Verification items for the finished model (mm, model axes). A direction names the side the tool comes from. Give positions to 0.01 mm unless a question says otherwise; leave off trailing zeros. Order: outer loops, then holes, each group sorted by start corner. A loop starts at its lowest first (then second) coordinate and runs counter-clockwise, first axis right, second up. Notation, with made-up numbers: (22, 60) -> (32, 60) arc R30 cw to (32, 98) -> close; hole circle Ø10 at (-14.75, -5). An arc over 180 degrees is marked (long way). Write each question's results on one line, items separated by ' | '. Start each with the question number.
1. Cross-section at C-C, the plane x = 12. Enter the section's corners in (y, z), then the cut area to 3 significant figures.
2. Cross-section at D-D, the plane x = -12.7. Enter the section's corners in (y, z), then the cut area to 3 significant figures.
3. Cross-section at A-A, the plane y = 0. Enter the section's corners in (x, z).
4. Cross-section at B-B, the plane z = 1.75. Enter the section's corners in (x, y), then the cut area to 3 significant figures.
5. Set-up check for faces 1 (the face through (0, 1.5, 1)), 2 (the face through (-11.746, 0.3, 1.479)), 3 (the face through (-9.066, -1.763, 1.521)): record each of +Z, -Z, +X, -X, +Y, -Y from which the full face is reachable in a straight line by a thin tool's end or side.
6. Material ranges on L1, parallel to Y at x = -12.7, z = 1.7; L2, parallel to X at y = 0.75, z = 1.4; L3, parallel to X at y = 0.5, z = 0.6, recorded low to high. Write a range as from..to.
7. Mould release check, pull along X, two halves, no side actions. Record for faces 4 (the face through (0, 0, 3)), 5 (the face through (-9.104, 1.778, 1.521)): +X half, -X half, draft (parallel to the pull), parting line (faces both ways), or undercut.
8. Depth check by flat-ended pin: pin 1 Ø2.5 at (x, y) = (-12.7, 0) entering from +Z; pin 2 Ø0.9 at (x, z) = (1.5, 2) entering from -Y. Enter the tip coordinate at first touch or a pass-through.
from build123d import *

# Parameters (mm, degrees)
SKETCH_1_R      = 1
EXTRUDE_1_DEPTH = 3
FILLET_1_R      = 3.81


with BuildPart() as part:
    # 스케치1 → 보스-돌출1 (new body)
    with BuildSketch(Plane.XY):
        with BuildLine():
            Line((-9.53772234, -1.5), (9.53772234, -1.5))
            ThreePointArc((9.53772234, -1.5), (16.2, 0), (9.53772234, 1.5))
            Line((9.53772234, 1.5), (-9.53772234, 1.5))
            ThreePointArc((-9.53772234, 1.5), (-16.2, 0), (-9.53772234, -1.5))
        make_face()
        with Locations((-12.7, 0)):
            Circle(SKETCH_1_R, mode=Mode.SUBTRACT)
        with Locations((12.7, 0)):
            Circle(SKETCH_1_R, mode=Mode.SUBTRACT)
    extrude(amount=EXTRUDE_1_DEPTH)

    # 필렛1
    fillet_1_edges = [part.edges().sort_by_distance(p)[0] for p in [
        (9.53772234, -1.5, 1.5),
        (-9.53772234, -1.5, 1.5),
        (-9.53772234, 1.5, 1.5),
        (9.53772234, 1.5, 1.5),
    ]]
    fillet(fillet_1_edges, radius=FILLET_1_R)


solid = part.part
Results below:
1) outline: (-3.43, 0) -> (-0.71, 0) -> (-0.71, 3) -> (-3.43, 3) -> close; (0.71, 0) -> (3.43, 0) -> (3.43, 3) -> (0.71, 3) -> close | area: 16.3 mm²
2) outline: (-3.5, 0) -> (-1, 0) -> (-1, 3) -> (-3.5, 3) -> close; (1, 0) -> (3.5, 0) -> (3.5, 3) -> (1, 3) -> close | area: 15.0 mm²
3) outline: (-16.2, 0) -> (-13.7, 0) -> (-13.7, 3) -> (-16.2, 3) -> close; (-11.7, 0) -> (11.7, 0) -> (11.7, 3) -> (-11.7, 3) -> close; (13.7, 0) -> (16.2, 0) -> (16.2, 3) -> (13.7, 3) -> close
4) outline: (-10.29, -2.54) arc R3.81 cw to (-7.68, -1.5) -> (7.68, -1.5) arc R3.81 cw to (10.29, -2.54) arc R3.5 ccw (long way) to (10.29, 2.54) arc R3.81 cw to (7.68, 1.5) -> (-7.68, 1.5) arc R3.81 cw to (-10.29, 2.54) arc R3.5 ccw (long way) to start; hole circle Ø2 at (-12.7, 0); hole circle Ø2 at (12.7, 0) | area: 128 mm²
5) face 1: +Z, -Z, +Y | face 2: +Z, -Z | face 3: +Z, -Z, -Y
6) L1: y = -3.5..-1, 1..3.5 | L2: x = -16.12..-13.36, -12.04..12.04, 13.36..16.12 | L3: x = -16.16..-13.57, -11.83..11.83, 13.57..16.16
7) face 4: draft | face 5: undercut
8) pin 1: stops at z = 3 | pin 2: stops at y = -1.5
